Source: three-view drawing plus pictorial views. Frame: mm from the lowest corner of the part. A direction names the side the tool comes from. Round coordinates to 2 decimals unless told otherwise and drop trailing zeros. Order: outer loops, then holes, each group sorted by start corner. A loop starts at its lowest first (then second) coordinate and runs counter-clockwise, first axis right, second up. Notation, with made-up numbers: M 25.25,70 L 58.25,70 A9 ccw 58.25,80 Z; hole C -18,36.5 d1. An arc over 180 degrees is marked long. Return JSON: item names as keys, results as strings. Group by question number.
Q1. Contact query for flat-ended pins moving along their axis: pin 1 (2.5 mm diameter, centred on x = 18.5, y = 3.5, fed in from -Z) (1 decimal); pin 2 (1 mm diameter, centred on x = 10.5, y = 4, fed in from +Z); pin 3 (2 mm diameter, centred on x = 19.5, y = 2, fed in from -Z); pin 4 (2 mm diameter, centred on x = 11, z = 5.5, fed in from -Y). Output: stop coordinate, or through.
Q2. Cut plane B-B on z = 2.5. Output: boundary loops of the cut face in (x, y), and give its area (3 significant figures).
Q3. Cut plane A-A on x = 18. Output: boundary loops of the cut face in (y, z).
Q4. Mould query, pull axis X, two halves, no side actions, for the marked faces 1, 2 and 3. Classes: released by +X, released by -X, zero draft, split by the parting line, or undercut.
Q5. Cut plane C-C on y = 3.15. Output: boundary loops of the cut face in (x, z), and give its area (3 significant figures).
Q6. Cut plane D-D on x = 4. Output: boundary loops of the cut face in (y, z) (3 decimals).
Q7. Ray query, probe 1 along Z at (x, y) = (12, 3.8); probe 2 along Z at (x, y) = (18.25, 0.5); probe 3 along X at (y, z) = (3.35, 6). Return the intervals inside material, ascending.
Q8. Access query for the marked faces 4, 5, 6 and 7. Directions: +Z, -Z, +X, -X, +Y, -Y. A direction counts if a zero-diameter tool reaches every point of the face in a straight line with its end or side. Return the directions, or none.
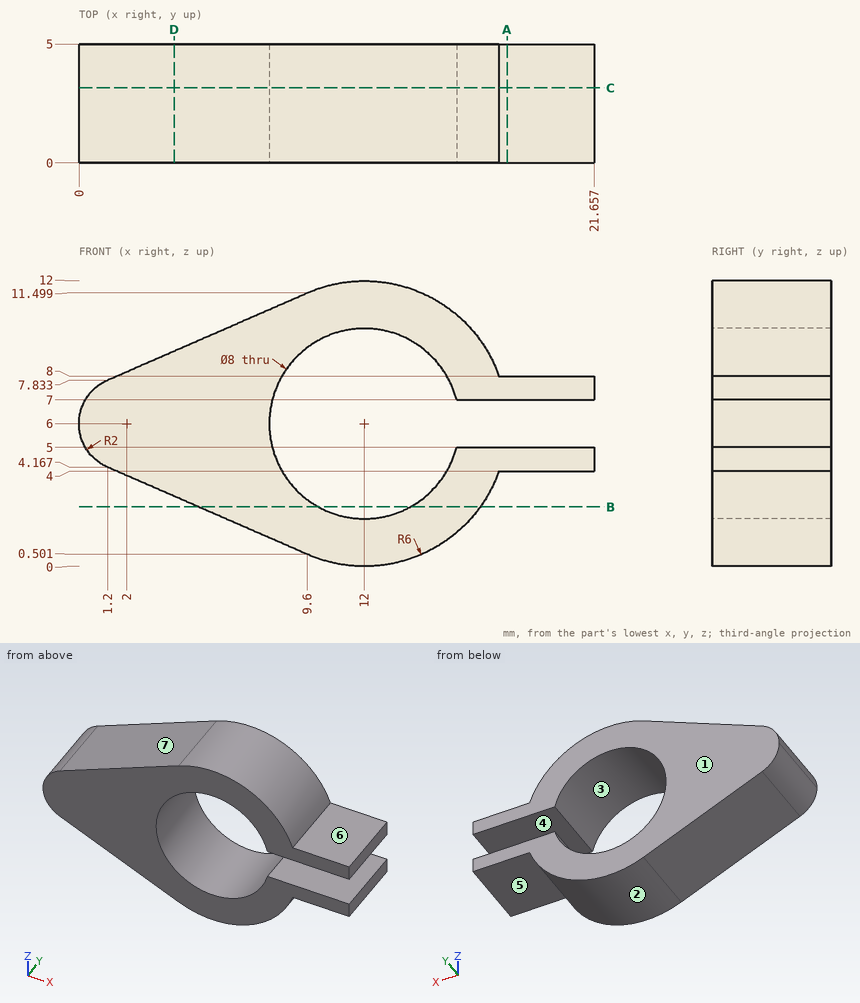
Result sheet:
{
 "1": {"pin 1": "stops at z = 3.1", "pin 2": "stops at z = 11.92", "pin 3": "stops at z = 4", "pin 4": "passes through"},
 "2": {"outline": "M 5.02,0 L 10.06,0 L 10.06,5 L 5.02,5 Z; M 13.94,0 L 16.87,0 L 16.87,5 L 13.94,5 Z", "area": "39.9 mm²"},
 "3": {"outline": "M 0,4 L 5,4 L 5,5 L 0,5 Z; M 0,7 L 5,7 L 5,8 L 0,8 Z"},
 "4": {"face 1": "zero draft", "face 2": "split by the parting line", "face 3": "undercut"},
 "5": {"outline": "M 1.2,4.17 L 9.6,0.5 A6 ccw 17.66,4 L 21.66,4 L 21.66,5 L 15.87,5 A4 cw long 15.87,7 L 21.66,7 L 21.66,8 L 17.66,8 A6 ccw 9.6,11.5 L 1.2,7.83 A2 ccw Z", "area": "103 mm²"},
 "6": {"outline": "M 0,2.945 L 5,2.945 L 5,9.055 L 0,9.055 Z"},
 "7": {"probe 1": "z = 0 to 2, 10 to 12", "probe 2": "z = 4 to 5, 7 to 8", "probe 3": "x = 0 to 8"},
 "8": {"face 4": "+X, +Y, -Y", "face 5": "-Z, +X, +Y, -Y", "face 6": "+Z, +X, +Y, -Y", "face 7": "+Z, -X, +Y, -Y"}
}
